Build history of the part. All positions in model axes, mm. A direction names the side the tool comes from. Give positions to 0.01 mm unless a question says otherwise; leave off trailing zeros. Order: outer loops, then holes, each group sorted by start corner. A loop starts at its lowest first (then second) coordinate and runs counter-clockwise, first axis right, second up. Notation, with made-up numbers: (77, 18) - (104, 18) arc R25 cw to (104, 46) - close; hole circle Ø1 at (-27.75, -35.75). An arc over 180 degrees is marked (long way). Use a Markdown table: item, result.
from build123d import *

# Parameters (mm, degrees)
FILLET1_R           = 10
SHELL1_T            = -2.7
SKETCH4_R           = 2
BOSS_EXTRUDE1_DEPTH = 10


with BuildPart() as part:
    # Sketch2 → Loft1 section 0
    with BuildSketch(Plane.XY.offset(27)):
        with BuildLine():
            Line((-54, 73.5), (54, 73.5))
            Line((54, 73.5), (54, -73.5))
            Line((54, -73.5), (-54, -73.5))
            Line((-54, -73.5), (-54, 73.5))
        make_face()
    # Sketch1 → Loft1 section 1
    with BuildSketch(Plane.XY):
        with BuildLine():
            Line((54, 73.5), (-54, 73.5))
            Line((-54, 73.5), (-54, -73.5))
            Line((-54, -73.5), (54, -73.5))
            Line((54, -73.5), (54, 73.5))
        make_face()
    loft()

    # Fillet1
    fillet1_edges = [part.edges().sort_by_distance(p)[0] for p in [
        (0, -73.5, 27),
        (-54, 0, 27),
        (0, 73.5, 27),
        (54, 0, 27),
        (54, 73.5, 13.5),
        (-54, 73.5, 13.5),
        (-54, -73.5, 13.5),
        (54, -73.5, 13.5),
    ]]
    fillet(fillet1_edges, radius=FILLET1_R)

    # Shell1
    shell1_openings = [part.faces().sort_by_distance(p)[0] for p in [
        (9.6e-08, -7.1e-08, 0),
    ]]
    offset(amount=SHELL1_T, openings=shell1_openings)

    # Sketch4 → Boss-Extrude1 (add)
    with BuildSketch(Plane(origin=(0, 50, 0), x_dir=(1, 0, 0), z_dir=(0, 1, 0))):
        with BuildLine():
            Line((57.194341554, 1.825338031), (54, 0))
            Line((54, 0), (54, -17))
            Line((54, -17), (59.613919523, -0.158241431))
            ThreePointArc((59.613919523, -0.158241431), (63.778881993, 7.3896911), (57.194341554, 1.825338031))
        make_face()
        with Locations(Location((61, 4, 0), (0, 0, 270))):
            Circle(SKETCH4_R, mode=Mode.SUBTRACT)
    boss_extrude1 = extrude(amount=BOSS_EXTRUDE1_DEPTH)

    # Mirror1: Boss-Extrude1 across plane
    add(boss_extrude1.mirror(Plane.ZX))


solid = part.part
1) Pin check, flat tips, straight feed: P1, Ø8, axis at y = -8.5, z = 21.5, coming from the +X side; P2, Ø5.5, axis at x = 59, z = 0.5, coming from the +Y side; P3, Ø9, axis at x = 60, z = 5, coming from the -Y side. Stop position of each tip, or through.
Computed:
| item | result |
|---|---|
| P1 | stops at x = 53.99 |
| P2 | stops at y = 60 |
| P3 | stops at y = -60 |
2) Tool access for faces 1 (the cylindrical face through (-0.616, -68.718, 22.105)), 2 (the flat face through (58, 50, 0)), 3 (the flat face through (58, 60, 0)), 4 (the flat face through (58, -60, 0)): list every direction of +Z, -Z, +X, -X, +Y, -Y with a clear straight run to the whole face (end or side of a thin tool).
Computed:
| item | result |
|---|---|
| face 1 | -Z |
| face 2 | +Z, -Z, +X |
| face 3 | +Z, -Z, +X, +Y |
| face 4 | +Z, -Z, +X, -Y |
3) Wall check: line 1 (Y direction, x = 18, z = 6.5); line 2 (X direction, y = -57, z = -4); line 3 (X direction, y = -42.5, z = 4). Give the ranges that are in metal, low to high. Write a range as from..to.
Computed:
| item | result |
|---|---|
| line 1 | y = -73.5..-70.8, 70.8..73.5 |
| line 2 | x = 56.62..59, 63..65.38 |
| line 3 | x = -54..-51.3, 51.3..54 |
4) Two-plate mould, pull along X, no slides. Class faces 5 (the flat face through (-1, 70.8, 8)), 6 (the flat face through (54, 62, 8)), 7 (the cylindrical face through (-51.15, 0.89, 23.99)), 8 (the flat face through (58, -50, 0)): +X half, -X half, draft (parallel to the pull), parting line (faces both ways), or undercut.
Computed:
| item | result |
|---|---|
| face 5 | undercut |
| face 6 | +X half |
| face 7 | -X half |
| face 8 | draft |
5) Slice it at C-C (y = 6). Write the cut outline in (x, z).
Computed:
| item | result |
|---|---|
| outline | (-54, 0) - (-51.3, 0) - (-51.3, 17) arc R7.3 cw to (-44, 24.3) - (44, 24.3) arc R7.3 cw to (51.3, 17) - (51.3, 0) - (54, 0) - (54, 17) arc R10 ccw to (44, 27) - (-44, 27) arc R10 ccw to (-54, 17) - close |
6) Slice it at B-B (x = 6.5). Write the cut outline in (y, z), and give its area (3 significant figures).
Computed:
| item | result |
|---|---|
| outline | (-73.5, 0) - (-70.8, 0) - (-70.8, 17) arc R7.3 cw to (-63.5, 24.3) - (63.5, 24.3) arc R7.3 cw to (70.8, 17) - (70.8, 0) - (73.5, 0) - (73.5, 17) arc R10 ccw to (63.5, 27) - (-63.5, 27) arc R10 ccw to (-73.5, 17) - close |
| area | 508 mm² |
7) Slice it at A-A (z = -4). Write the cut outline in (x, y), and give its area (3 significant figures).
Computed:
| item | result |
|---|---|
| outline | (56.62, -60) - (59, -60) - (59, -50) - (56.62, -50) - close; (56.62, 50) - (59, 50) - (59, 60) - (56.62, 60) - close; (63, -60) - (65.38, -60) - (65.38, -50) - (63, -50) - close; (63, 50) - (65.38, 50) - (65.38, 60) - (63, 60) - close |
| area | 95.3 mm² |
